from build123d import *

# Parameters (mm, degrees)
BOSS_EXTRUDE1_DEPTH = 8


with BuildPart() as part:
    # Model → Boss-Extrude1 (new body)
    with BuildSketch(Plane.XY):
        with BuildLine():
            Line((-65, -10), (-65, -19.5))
            ThreePointArc((-65, -19.5), (-64.853553391, -19.853553391), (-64.5, -20))
            Line((-64.5, -20), (-38.2, -20))
            ThreePointArc((-38.2, -20), (-38.058578644, -19.941421356), (-38, -19.8))
            Line((-38, -19.8), (-38, -15.2))
            ThreePointArc((-38, -15.2), (-38.058578644, -15.058578644), (-38.2, -15))
            Line((-38.2, -15), (-39.8, -15))
            ThreePointArc((-39.8, -15), (-39.941421356, -14.941421356), (-40, -14.8))
            Line((-40, -14.8), (-40, -10.2))
            ThreePointArc((-40, -10.2), (-39.941421356, -10.058578644), (-39.8, -10))
            Line((-39.8, -10), (-38.2, -10))
            ThreePointArc((-38.2, -10), (-38.058578644, -9.941421356), (-38, -9.8))
            Line((-38, -9.8), (-38, -4.5))
            ThreePointArc((-38, -4.5), (-37.853553391, -4.146446609), (-37.5, -4))
            Line((-37.5, -4), (-32.5, -4))
            ThreePointArc((-32.5, -4), (-32.146446609, -4.146446609), (-32, -4.5))
            Line((-32, -4.5), (-32, -9.8))
            ThreePointArc((-32, -9.8), (-31.941421356, -9.941421356), (-31.8, -10))
            Line((-31.8, -10), (-30.2, -10))
            ThreePointArc((-30.2, -10), (-30.058578644, -10.058578644), (-30, -10.2))
            Line((-30, -10.2), (-30, -14.8))
            ThreePointArc((-30, -14.8), (-30.058578644, -14.941421356), (-30.2, -15))
            Line((-30.2, -15), (-31.8, -15))
            ThreePointArc((-31.8, -15), (-31.941421356, -15.058578644), (-32, -15.2))
            Line((-32, -15.2), (-32, -19.8))
            ThreePointArc((-32, -19.8), (-31.941421356, -19.941421356), (-31.8, -20))
            Line((-31.8, -20), (-10, -20))
            Line((-10, -20), (-10, -35))
            Line((-10, -35), (10, -35))
            Line((10, -35), (10, -20))
            Line((10, -20), (31.8, -20))
            ThreePointArc((31.8, -20), (31.941421356, -19.941421356), (32, -19.8))
            Line((32, -19.8), (32, -15.2))
            ThreePointArc((32, -15.2), (31.941421356, -15.058578644), (31.8, -15))
            Line((31.8, -15), (30.2, -15))
            ThreePointArc((30.2, -15), (30.058578644, -14.941421356), (30, -14.8))
            Line((30, -14.8), (30, -10.2))
            ThreePointArc((30, -10.2), (30.058578644, -10.058578644), (30.2, -10))
            Line((30.2, -10), (31.8, -10))
            ThreePointArc((31.8, -10), (31.941421356, -9.941421356), (32, -9.8))
            Line((32, -9.8), (32, -4.5))
            ThreePointArc((32, -4.5), (32.146446609, -4.146446609), (32.5, -4))
            Line((32.5, -4), (37.5, -4))
            ThreePointArc((37.5, -4), (37.853553391, -4.146446609), (38, -4.5))
            Line((38, -4.5), (38, -9.8))
            ThreePointArc((38, -9.8), (38.058578644, -9.941421356), (38.2, -10))
            Line((38.2, -10), (39.8, -10))
            ThreePointArc((39.8, -10), (39.941421356, -10.058578644), (40, -10.2))
            Line((40, -10.2), (40, -14.8))
            ThreePointArc((40, -14.8), (39.941421356, -14.941421356), (39.8, -15))
            Line((39.8, -15), (38.2, -15))
            ThreePointArc((38.2, -15), (38.058578644, -15.058578644), (38, -15.2))
            Line((38, -15.2), (38, -19.8))
            ThreePointArc((38, -19.8), (38.058578644, -19.941421356), (38.2, -20))
            Line((38.2, -20), (64.5, -20))
            ThreePointArc((64.5, -20), (64.853553391, -19.853553391), (65, -19.5))
            Line((65, -19.5), (65, -10))
            ThreePointArc((65, -10), (62.071067812, -2.928932188), (55, 0))
            Line((55, 0), (-55, 0))
            ThreePointArc((-55, 0), (-62.071067812, -2.928932188), (-65, -10))
        make_face()
    extrude(amount=BOSS_EXTRUDE1_DEPTH)


solid = part.part
Input: part model. Units: mm. Frame: model coordinates. A direction names the side the tool comes from. Coordinates: 2 decimals unless noted, no trailing zeros. Loops run counter-clockwise (first coordinate to the right, second up) from the corner with the lowest first, then second, coordinate; pieces in that order, holes last.
(1) Material intervals for probe 1 along X at (y, z) = (-17, 2.5); probe 2 along X at (y, z) = (-10.5, 6.5); probe 3 along Y at (x, z) = (38.5, 6.5), sorted ascending.
(2) Section D-D on y = -22. Return the cut outline in (x, z), then the cut area to 3 significant figures.
(3) Set-up query: faces 5 (the face through (-52, -20, 4)), 6 (the face through (-32, -17, 4)), 7 (the face through (10, -28, 4)), 8 (the face through (-30, -12, 4)), 9 (the face through (-1, -9, 8)). Return all of +Z, -Z, +X, -X, +Y, -Y with unobstructed straight access to the full face (end or side cutting, diameter ignored); none if empty.
(4) Section C-C on y = -7. Return the cut outline in (x, z).
(5) First-contact query: pin 1 Ø1.8 at (x, z) = (-39, 4) entering from -Y; pin 2 Ø4 at (y, z) = (-8.5, 5) entering from -X; pin 3 Ø8 at (x, y) = (33.5, -25.5) entering from +Z; pin 4 Ø2.5 at (x, z) = (-34, 2.5) entering from -Y. Flat tips, straight axial feed; report the tip coordinate or a pass-through.
(6) Pull-direction query (X, two-part tool) for faces 1 (the face through (1, 0, 4)), 2 (the face through (-40, -13, 4)), 3 (the face through (62.15, -3.01, 3.94)), 4 (the face through (-38, -7, 4)); classes: released by +X, released by -X, zero draft, split by the parting line, or undercut.
(7) Section A-A on y = -12.5. Return the cut outline in (x, z).
(8) Section B-B on x = -23. Return the cut outline in (y, z).
Data:
1. probe 1: x = -65 to -38, -32 to 32, 38 to 65
1. probe 2: x = -65 to -40, -30 to 30, 40 to 65
1. probe 3: y = -20 to -15, -10 to 0
2. outline: (-10, 0) - (10, 0) - (10, 8) - (-10, 8) - close
2. area: 160 mm2
3. face 5: +Z, -Z, -X, -Y
3. face 6: +Z, -Z, -Y
3. face 7: +Z, -Z, +X, -Y
3. face 8: +Z, -Z
3. face 9: +Z, +X, -X, +Y, -Y
4. outline: (-64.54, 0) - (-38, 0) - (-38, 8) - (-64.54, 8) - close; (-32, 0) - (32, 0) - (32, 8) - (-32, 8) - close; (38, 0) - (64.54, 0) - (64.54, 8) - (38, 8) - close
5. pin 1: stops at y = -20
5. pin 2: stops at x = -65
5. pin 3: passes through
5. pin 4: stops at y = -4
6. face 1: zero draft
6. face 2: undercut
6. face 3: released by +X
6. face 4: undercut
7. outline: (-65, 0) - (-40, 0) - (-40, 8) - (-65, 8) - close; (-30, 0) - (30, 0) - (30, 8) - (-30, 8) - close; (40, 0) - (65, 0) - (65, 8) - (40, 8) - close
8. outline: (-20, 0) - (0, 0) - (0, 8) - (-20, 8) - close
